Source: CAD feature listing. Evaluate the final solid. Frame: model axes, mm. A direction names the side the tool comes from. Give positions to 0.01 mm unless a question says otherwise; leave off trailing zeros. Write each loop counter-clockwise with the first axis right and the second up, starting at its lowest first coordinate (ties: lowest second). Pieces come first, ordered by that corner, then holes. Notation, with made-up numbers: (75, -12) -> (124, -12) arc R13 cw to (124, -7) -> close; hole circle Ø5 at (43.5, 36). An arc over 180 degrees is marked (long way). Answer as a JSON object with one key per item and string values. Group by question number.
Item 1: Ray query, probe 1 along X at (y, z) = (-0.5, 38.5); probe 2 along Z at (x, y) = (150.5, -22); probe 3 along Z at (x, y) = (21, 4). Return the intervals inside material, ascending. Write a range as from..to.
Item 2: First-contact query: pin 1 Ø5 at (y, z) = (-6, 75) entering from -X; pin 2 Ø10 at (x, y) = (142, 0) entering from +Z; pin 3 Ø6 at (y, z) = (5, 71) entering from +X. Flat tips, straight axial feed; report the tip coordinate or a pass-through.
Item 3: Pull-direction query (Z, two-part tool) for faces 1 (the face through (175, 0, 0)), 2 (the face through (-181, 6, 5)), 3 (the face through (-168.07, -2.87, 28.63)), 4 (the face through (-1.177, 0.33, 107.493)); classes: pulls with the +Z half, pulls with the -Z half, needs draft (parallel to the pull), parting line crosses it, or undercut.
Item 4: Section query B-B on z = 35.5. Return the cut outline in (x, y).
Item 5: Section query C-C on x = 55.5. Return the cut outline in (y, z), plus the area to 3 significant figures.
Item 6: Section query A-A on y = -13.5. Return the cut outline in (x, z).
Item 7: Access query for faces 5 (the face through (-175, 0, 0)), 6 (the face through (168.07, -2.87, 28.63)). Directions: +Z, -Z, +X, -X, +Y, -Y. A direction counts if a zero-diameter tool reaches every point of the face in a straight line with its end or side. Return the directions, or none.
from build123d import *

# Parameters (mm, degrees)
SKETCH1_W           = 50
SKETCH1_H           = 50
BOSS_EXTRUDE1_DEPTH = 5
SWEEP1_PROFILE_R    = 7.5
FILLET1_R           = 4


with BuildPart() as part:
    # Sketch1 → Boss-Extrude1 (new body)
    with BuildSketch(Plane.XY):
        with Locations((-175, 0)):
            Rectangle(SKETCH1_W, SKETCH1_H)
    extrude(amount=BOSS_EXTRUDE1_DEPTH)

    # Sweep1: sweep along a path in Sketch2
    with BuildLine(Plane(origin=(0, 0, 0), x_dir=(1, 0, 0), z_dir=(0, 1, 0))) as sweep1_path:
        Line((-175, -5), (-175, -51.606145517))
        ThreePointArc((-175, -51.606145517), (-171.61776041, -62.734938755), (-162.614996105, -70.099707486))
        Line((-162.614996105, -70.099707486), (-95.48773854, -97.740342954))
        ThreePointArc((-95.48773854, -97.740342954), (-89.887173245, -99.42966436), (-84.065244382, -100))
        Line((-84.065244382, -100), (0, -100))
    # Sweep1 profile (on start of the path) → Sweep1 (sweep)
    with BuildSketch(Plane(origin=(-175, 0, 5), x_dir=(1, 0, 0), z_dir=(0, 0, 1))):
        Circle(SWEEP1_PROFILE_R)
    sweep(path=sweep1_path.line)

    # Fillet1
    fillet1_edges = [part.edges().sort_by_distance(p)[0] for p in [
        (-150, -25, 2.5),
        (-200, -25, 2.5),
        (-200, 25, 2.5),
        (-150, 25, 2.5),
    ]]
    fillet(fillet1_edges, radius=FILLET1_R)

    # Mirror1: part across plane


with BuildPart() as part_1:
    add(part.part)
    add(part.part.mirror(Plane(origin=(0, 0, 0), x_dir=(0, 0, 1), z_dir=(1, 0, 0))))


solid = part_1.part
Worked answers:
{
 "1": {"probe 1": "-182.48..-167.52, 167.52..182.48", "probe 2": "0..5", "probe 3": "93.66..106.34"},
 "2": {"pin 1": "x = -169.79", "pin 2": "z = 88.76", "pin 3": "x = 175.7"},
 "3": {"face 1": "pulls with the -Z half", "face 2": "undercut", "face 3": "undercut", "face 4": "parting line crosses it"},
 "4": {"outline": "circle Ø15 at (-175, 0); circle Ø15 at (175, 0)"},
 "5": {"outline": "circle Ø15 at (0, 100)", "area": "177 mm^2"},
 "6": {"outline": "(-200, 0) -> (-150, 0) -> (-150, 5) -> (-200, 5) -> close; (150, 0) -> (200, 0) -> (200, 5) -> (150, 5) -> close"},
 "7": {"face 5": "-Z, +X, -X, +Y, -Y", "face 6": "none"}
}
